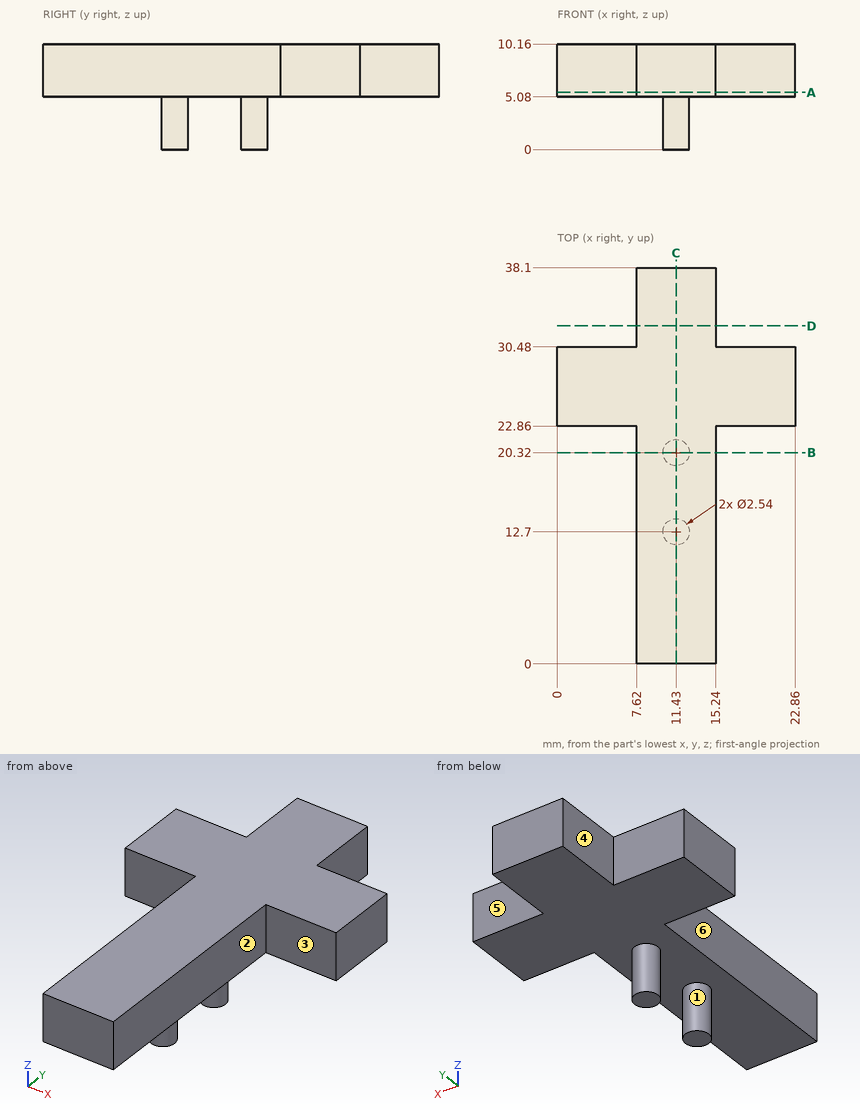
Source: three-view drawing plus pictorial views. Frame: mm from the lowest corner of the part. A direction names the side the tool comes from. Coordinates: 2 decimals unless noted, no trailing zeros. Loops run counter-clockwise (first coordinate to the right, second up) from the corner with the lowest first, then second, coordinate; pieces in that order, holes last. Notation, with made-up numbers: (49, 27.25) -> (89, 27.25) arc R18 cw to (89, 61.25) -> close; hole circle Ø2 at (8.5, -2). An arc over 180 degrees is marked (long way). Write each question's results on one line, items separated by ' | '. Start each with the question number.
Q1. Ray query, line 1 (Y direction, x = 21.5, z = 7); line 2 (X direction, y = 36, z = 6); line 3 (Z direction, x = 11.75, y = 4). Return the intervals inside material, ascending. Write a range as from..to.
Q2. Reachability of the marked faces 4, 5 and 6 from +Z, -Z, +X, -X, +Y, -Y: full face, straight path, thin tool, end or side. Return the list, or none.
Q3. Section D-D, the plane y = 32.5. Return the cut outline in (x, z), plus the area to 3 significant figures.
Q4. Section C-C, the plane x = 11.43. Return the cut outline in (y, z), plus the area to 3 significant figures.
Q5. Section B-B, the plane y = 20.32. Return the cut outline in (x, z).
Q6. Section A-A, the plane z = 5.5. Return the cut outline in (x, y), plus the area to 3 significant figures.
Q7. Pin query (flat end, axial travel): pin 1 (4 mm diameter, centred on x = 3.5, z = 7.5, fed in from +Y); pin 2 (5.5 mm diameter, centred on y = 34, z = 7, fed in from -X); pin 3 (4 mm diameter, centred on y = 6, z = 7, fed in from +X). Return the tip coordinate at first contact, or that it passes through.
Q8. Pull-direction query (Y, two-part tool) for the marked faces 1, 2 and 3; classes: released by +Y, released by -Y, zero draft, split by the parting line, or undercut.
Found:
1) line 1: 22.86..30.48 | line 2: 7.62..15.24 | line 3: 5.08..10.16
2) face 4: +Z, -Z, -X, +Y | face 5: +Z, -Z, +X, +Y | face 6: +Z, -Z, -X, -Y
3) outline: (7.62, 5.08) -> (15.24, 5.08) -> (15.24, 10.16) -> (7.62, 10.16) -> close | area: 38.7 mm2
4) outline: (0, 5.08) -> (11.43, 5.08) -> (11.43, 0) -> (13.97, 0) -> (13.97, 5.08) -> (19.05, 5.08) -> (19.05, 0) -> (21.59, 0) -> (21.59, 5.08) -> (38.1, 5.08) -> (38.1, 10.16) -> (0, 10.16) -> close | area: 219 mm2
5) outline: (7.62, 5.08) -> (10.16, 5.08) -> (10.16, 0) -> (12.7, 0) -> (12.7, 5.08) -> (15.24, 5.08) -> (15.24, 10.16) -> (7.62, 10.16) -> close
6) outline: (0, 22.86) -> (7.62, 22.86) -> (7.62, 0) -> (15.24, 0) -> (15.24, 22.86) -> (22.86, 22.86) -> (22.86, 30.48) -> (15.24, 30.48) -> (15.24, 38.1) -> (7.62, 38.1) -> (7.62, 30.48) -> (0, 30.48) -> close | area: 406 mm2
7) pin 1: y = 30.48 | pin 2: x = 7.62 | pin 3: x = 15.24
8) face 1: undercut | face 2: zero draft | face 3: released by -Y
